Check sheet for the modelled part. Datum: model origin and axes. Units: mm. A direction names the side the tool comes from. Round coordinates to 2 decimals unless told otherwise and drop trailing zeros. Order: outer loops, then holes, each group sorted by start corner. A loop starts at its lowest first (then second) coordinate and runs counter-clockwise, first axis right, second up.
```python
from build123d import *

# Parameters (mm, degrees)
SKETCH_2_W           = 60
SKETCH_2_H           = 60
EXTRUDE_1_DEPTH      = 3
SKETCH_6_R           = 1.5
CUT_EXTRUDE_2_DEPTH  = 3
EXTRUDE_START        = -30
EXTRUDE_2_DEPTH      = 30
EXTRUDE_START_2      = 30
EXTRUDE_3_DEPTH      = 30
CUT_EXTRUDE_START    = 13
SKETCH_9_W           = 10
SKETCH_9_H           = 10
CUT_EXTRUDE_3_DEPTH  = 10
CUT_EXTRUDE_START_2  = -15
SKETCH_10_W          = 5
SKETCH_10_H          = 5
CUT_EXTRUDE_4_DEPTH  = 5
CUT_EXTRUDE_START_3  = 10
SKETCH_11_W          = 5
SKETCH_11_H          = 5
CUT_EXTRUDE_5_DEPTH  = 5
EXTRUDE_5_DEPTH      = 1.6
EXTRUDE_START_3      = -1.6
SKETCH_17_W          = 28
SKETCH_17_H          = 8
SKETCH_17_W_2        = 8
SKETCH_17_H_2        = 28
EXTRUDE_6_DEPTH      = 2
SKETCH_21_R          = 12.5
EXTRUDE_8_DEPTH      = 4
CUT_EXTRUDE_START_4  = -4
SKETCH_22_R          = 1.5
CUT_EXTRUDE_6_DEPTH  = 4
EXTRUDE_START_4      = -4
SKETCH_23_R          = 1.5
EXTRUDE_9_DEPTH      = 4
EXTRUDE_START_5      = -3.6
SKETCH_24_W          = 8
SKETCH_24_H          = 28
SKETCH_24_W_2        = 28
SKETCH_24_H_2        = 8
EXTRUDE_10_DEPTH     = 0.4
EXTRUDE_START_6      = 3
SKETCH_25_W          = 10
SKETCH_25_H          = 3
SKETCH_25_W_2        = 3
SKETCH_25_H_2        = 10
EXTRUDE_11_DEPTH     = 10
SKETCH_26_W          = 55
SKETCH_26_H          = 5
SKETCH_26_W_2        = 5
SKETCH_26_H_2        = 55
EXTRUDE_12_DEPTH     = 10
CUT_EXTRUDE_START_5  = -30
CUT_EXTRUDE_7_DEPTH  = 5
CUT_EXTRUDE_START_6  = 25
CUT_EXTRUDE_8_DEPTH  = 5
CUT_EXTRUDE_START_7  = 3
SKETCH_31_R          = 1
CUT_EXTRUDE_10_DEPTH = 3
CUT_EXTRUDE_11_DEPTH = 4
CUT_EXTRUDE_12_DEPTH = 13
SKETCH_34_W          = 20
SKETCH_34_H          = 20
CUT_EXTRUDE_14_DEPTH = 3
SKETCH_35_W          = 20
SKETCH_35_H          = 10
EXTRUDE_14_DEPTH     = 5
SKETCH_36_W          = 20
SKETCH_36_H          = 10
EXTRUDE_15_DEPTH     = 5
EXTRUDE_16_DEPTH     = 5
EXTRUDE_18_DEPTH     = 5
EXTRUDE_19_DEPTH     = 4
CUT_EXTRUDE_START_8  = -22
CUT_EXTRUDE_15_DEPTH = 44
CUT_EXTRUDE_16_DEPTH = 44
FILLET_1_R           = 5
FILLET_2_R           = 3


# Some blends are built 0.0001 mm under size
with BuildPart() as part:
    # 草图2 → 凸台-拉伸1 (new body)
    with BuildSketch(Plane(origin=(0, 0, 0), x_dir=(1, 0, 0), z_dir=(0, 1, 0))):
        Rectangle(SKETCH_2_W, SKETCH_2_H)
    extrude(amount=EXTRUDE_1_DEPTH)

    # 草图6 → 切除-拉伸2 (cut)
    with BuildSketch(Plane(origin=(0, 0, 0), x_dir=(1, 0, 0), z_dir=(0, 1, 0))):
        with Locations(Location((0, -7, 0), (0, 0, 270))):
            Circle(SKETCH_6_R)
        with Locations(Location((7, 0, 0), (0, 0, 270))):
            Circle(SKETCH_6_R)
        with Locations(Location((0, 7, 0), (0, 0, 270))):
            Circle(SKETCH_6_R)
        with Locations(Location((-7, 0, 0), (0, 0, 270))):
            Circle(SKETCH_6_R)
    extrude(amount=CUT_EXTRUDE_2_DEPTH, mode=Mode.SUBTRACT)

    # 草图7 → 凸台-拉伸2 (add)
    with BuildSketch(Plane.XY.offset(EXTRUDE_START)):
        Polygon((-15, 3), (-15, 8), (-20, 8), (-20, 13), (-10, 13), (-10, 3), align=None)
        Polygon((10, 3), (15, 3), (15, 8), (20, 8), (20, 13), (10, 13), align=None)
    extrude(amount=EXTRUDE_2_DEPTH)

    # 草图8 → 凸台-拉伸3 (add)
    with BuildSketch(Plane(origin=(0, 0, 0), x_dir=(0, 0, -1), z_dir=(1, 0, 0)).offset(EXTRUDE_START_2)):
        Polygon((-15, 3), (-15, 8), (-20, 8), (-20, 13), (-10, 13), (-10, 3), align=None)
        Polygon((10, 3), (15, 3), (15, 8), (20, 8), (20, 13), (10, 13), align=None)
    extrude(amount=-EXTRUDE_3_DEPTH)

    # 草图9 → 切除-拉伸3 (cut)
    with BuildSketch(Plane(origin=(0, 0, 0), x_dir=(1, 0, 0), z_dir=(0, 1, 0)).offset(CUT_EXTRUDE_START)):
        with Locations((25, 15)):
            Rectangle(SKETCH_9_W, SKETCH_9_H)
        with Locations((15, 25)):
            Rectangle(SKETCH_9_W, SKETCH_9_H)
    extrude(amount=-CUT_EXTRUDE_3_DEPTH, mode=Mode.SUBTRACT)

    # 草图10 → 切除-拉伸4 (cut)
    with BuildSketch(Plane.XY.offset(CUT_EXTRUDE_START_2)):
        with Locations((17.5, 5.5)):
            Rectangle(SKETCH_10_W, SKETCH_10_H)
    extrude(amount=CUT_EXTRUDE_4_DEPTH, mode=Mode.SUBTRACT)

    # 草图11 → 切除-拉伸5 (cut)
    with BuildSketch(Plane(origin=(0, 0, 0), x_dir=(0, 0, -1), z_dir=(1, 0, 0)).offset(CUT_EXTRUDE_START_3)):
        with Locations((17.5, 5.5)):
            Rectangle(SKETCH_11_W, SKETCH_11_H)
    extrude(amount=CUT_EXTRUDE_5_DEPTH, mode=Mode.SUBTRACT)

    # 草图16 → 凸台-拉伸5 (add)
    with BuildSketch(Plane(origin=(0, 0, 0), x_dir=(1, 0, 0), z_dir=(0, 1, 0))):
        Polygon((-10, -25), (15, -25), (15, -30), (18, -30), (18, -22), (-10, -22), align=None)
        Polygon((-22, 18), (-22, -10), (-25, -10), (-25, 15), (-30, 15), (-30, 18), align=None)
    extrude(amount=-EXTRUDE_5_DEPTH)

    # 草图17 → 凸台-拉伸6 (add)
    with BuildSketch(Plane(origin=(0, 0, 0), x_dir=(1, 0, 0), z_dir=(0, 1, 0)).offset(EXTRUDE_START_3)):
        with Locations((4, -26)):
            Rectangle(SKETCH_17_W, SKETCH_17_H)
        with Locations((-26, 4)):
            Rectangle(SKETCH_17_W_2, SKETCH_17_H_2)
    extrude(amount=-EXTRUDE_6_DEPTH)

    # 草图21 → 凸台-拉伸8 (add)
    with BuildSketch(Plane(origin=(0, 0, 0), x_dir=(1, 0, 0), z_dir=(0, 1, 0))):
        with Locations(Location((0, 0, 0), (0, 0, 270))):
            Circle(SKETCH_21_R)
    extrude(amount=-EXTRUDE_8_DEPTH)

    # 草图22 → 切除-拉伸6 (cut)
    with BuildSketch(Plane(origin=(0, 0, 0), x_dir=(1, 0, 0), z_dir=(0, 1, 0)).offset(CUT_EXTRUDE_START_4)):
        with Locations(Location((7, 0, 0), (0, 0, 270))):
            Circle(SKETCH_22_R)
        with Locations(Location((0, -7, 0), (0, 0, 270))):
            Circle(SKETCH_22_R)
        with Locations(Location((-7, 0, 0), (0, 0, 270))):
            Circle(SKETCH_22_R)
        with Locations(Location((0, 7, 0), (0, 0, 270))):
            Circle(SKETCH_22_R)
    extrude(amount=CUT_EXTRUDE_6_DEPTH, mode=Mode.SUBTRACT)

    # 草图23 → 凸台-拉伸9 (add)
    with BuildSketch(Plane(origin=(0, 0, 0), x_dir=(1, 0, 0), z_dir=(0, 1, 0)).offset(EXTRUDE_START_4)):
        Polygon((22, -18), (18, -22), (-10, -22), (-22, -10), (-22, 18), (-18, 22), (-18, 30), (18, 30), (18, 22), (22, 18), (30, 18), (30, -18), align=None)
        with Locations(Location((0, 7, 0), (0, 0, 270))):
            Circle(SKETCH_23_R, mode=Mode.SUBTRACT)
        with Locations(Location((7, 0, 0), (0, 0, 270))):
            Circle(SKETCH_23_R, mode=Mode.SUBTRACT)
        with Locations(Location((-7, 0, 0), (0, 0, 270))):
            Circle(SKETCH_23_R, mode=Mode.SUBTRACT)
        with Locations(Location((0, -7, 0), (0, 0, 270))):
            Circle(SKETCH_23_R, mode=Mode.SUBTRACT)
    extrude(amount=EXTRUDE_9_DEPTH)

    # 草图24 → 凸台-拉伸10 (add)
    with BuildSketch(Plane(origin=(0, 0, 0), x_dir=(1, 0, 0), z_dir=(0, 1, 0)).offset(EXTRUDE_START_5)):
        with Locations((-26, 4)):
            Rectangle(SKETCH_24_W, SKETCH_24_H)
        with Locations((4, -26)):
            Rectangle(SKETCH_24_W_2, SKETCH_24_H_2)
    extrude(amount=-EXTRUDE_10_DEPTH)

    # 草图25 → 凸台-拉伸11 (add)
    with BuildSketch(Plane(origin=(0, 0, 0), x_dir=(1, 0, 0), z_dir=(0, 1, 0)).offset(EXTRUDE_START_6)):
        with Locations((-15, -1.5)):
            Rectangle(SKETCH_25_W, SKETCH_25_H)
        with Locations((-1.5, -15)):
            Rectangle(SKETCH_25_W_2, SKETCH_25_H_2)
    extrude(amount=EXTRUDE_11_DEPTH)

    # 草图26 → 凸台-拉伸12 (add)
    with BuildSketch(Plane(origin=(0, 0, 0), x_dir=(1, 0, 0), z_dir=(0, 1, 0)).offset(EXTRUDE_START_6)):
        with Locations((2.5, -27.5)):
            Rectangle(SKETCH_26_W, SKETCH_26_H)
        with Locations((-27.5, 2.5)):
            Rectangle(SKETCH_26_W_2, SKETCH_26_H_2)
        with Locations((-27.5, -27.5)):
            Rectangle(SKETCH_26_W_2, SKETCH_26_H)
    extrude(amount=EXTRUDE_12_DEPTH)

    # 草图27 → 切除-拉伸7 (cut)
    with BuildSketch(Plane(origin=(0, 0, 0), x_dir=(0, 0, -1), z_dir=(1, 0, 0)).offset(CUT_EXTRUDE_START_5)):
        with BuildLine():
            Line((22.5, 6), (-22.5, 6))
            ThreePointArc((-22.5, 6), (-24.5, 8), (-22.5, 10))
            Line((-22.5, 10), (22.5, 10))
            ThreePointArc((22.5, 10), (24.5, 8), (22.5, 6))
        make_face()
    extrude(amount=CUT_EXTRUDE_7_DEPTH, mode=Mode.SUBTRACT)

    # 草图28 → 切除-拉伸8 (cut)
    with BuildSketch(Plane.XY.offset(CUT_EXTRUDE_START_6)):
        with BuildLine():
            Line((-22.5, 10), (22.5, 10))
            ThreePointArc((22.5, 10), (24.5, 8), (22.5, 6))
            Line((22.5, 6), (-22.5, 6))
            ThreePointArc((-22.5, 6), (-24.5, 8), (-22.5, 10))
        make_face()
    extrude(amount=CUT_EXTRUDE_8_DEPTH, mode=Mode.SUBTRACT)

    # 草图31 → 切除-拉伸10 (cut)
    with BuildSketch(Plane(origin=(0, 0, 0), x_dir=(1, 0, 0), z_dir=(0, 1, 0)).offset(CUT_EXTRUDE_START_7)):
        with Locations(Location((-20, -20, 0), (0, 0, 270))):
            Circle(SKETCH_31_R)
    extrude(amount=-CUT_EXTRUDE_10_DEPTH, mode=Mode.SUBTRACT)

    # 草图32 → 切除-拉伸11 (cut)
    with BuildSketch(Plane(origin=(0, 0, 0), x_dir=(1, 0, 0), z_dir=(0, 1, 0))):
        Polygon((30, 30), (30, 25), (25, 30), align=None)
    extrude(amount=CUT_EXTRUDE_11_DEPTH, mode=Mode.SUBTRACT)

    # 草图33 → 切除-拉伸12 (cut)
    with BuildSketch(Plane(origin=(0, 0, 0), x_dir=(1, 0, 0), z_dir=(0, 1, 0))):
        Polygon((-30, -30), (-27, -30), (-30, -27), align=None)
    extrude(amount=CUT_EXTRUDE_12_DEPTH, mode=Mode.SUBTRACT)

    # 草图34 → 切除-拉伸14 (cut)
    with BuildSketch(Plane(origin=(0, 0, 0), x_dir=(1, 0, 0), z_dir=(0, 1, 0)).offset(CUT_EXTRUDE_START_7)):
        Rectangle(SKETCH_34_W, SKETCH_34_H)
    extrude(amount=-CUT_EXTRUDE_14_DEPTH, mode=Mode.SUBTRACT)

    # 草图35 → 凸台-拉伸14 (add)
    with BuildSketch(Plane(origin=(0, 0, 0), x_dir=(0, 0, -1), z_dir=(1, 0, 0)).offset(EXTRUDE_START_2)):
        with Locations((0, 8)):
            Rectangle(SKETCH_35_W, SKETCH_35_H)
    extrude(amount=-EXTRUDE_14_DEPTH)

    # 草图36 → 凸台-拉伸15 (add)
    with BuildSketch(Plane.XY.offset(EXTRUDE_START)):
        with Locations((0, 8)):
            Rectangle(SKETCH_36_W, SKETCH_36_H)
    extrude(amount=EXTRUDE_15_DEPTH)

    # 草图37 → 凸台-拉伸16 (add)
    with BuildSketch(Plane.XY.offset(EXTRUDE_START)):
        Polygon((10, 3), (10, 13), (20, 13), (20, 8), (15, 8), (15, 3), align=None)
    extrude(amount=EXTRUDE_16_DEPTH)

    # 草图38 → 凸台-拉伸18 (add)
    with BuildSketch(Plane(origin=(0, 0, 0), x_dir=(0, 0, -1), z_dir=(1, 0, 0)).offset(EXTRUDE_START_2)):
        Polygon((10, 13), (20, 13), (20, 8), (15, 8), (15, 3), (10, 3), align=None)
    extrude(amount=-EXTRUDE_18_DEPTH)

    # 草图40 → 凸台-拉伸19 (add)
    with BuildSketch(Plane(origin=(0, 0, 0), x_dir=(1, 0, 0), z_dir=(0, 1, 0))):
        Polygon((-30, 18), (-18, 30), (-18, 22), (-22, 18), align=None)
        Polygon((18, 30), (30, 18), (22, 18), (18, 22), align=None)
        Polygon((30, -18), (18, -30), (18, -22), (22, -18), align=None)
    extrude(amount=-EXTRUDE_19_DEPTH)

    # 草图41 → 切除-拉伸15 (cut)
    with BuildSketch(Plane.XY.offset(CUT_EXTRUDE_START_8)):
        Polygon((30, 0), (26, -4), (30, -4), align=None)
    extrude(amount=CUT_EXTRUDE_15_DEPTH, mode=Mode.SUBTRACT)

    # 草图42 → 切除-拉伸16 (cut)
    with BuildSketch(Plane(origin=(0, 0, 0), x_dir=(0, 0, -1), z_dir=(1, 0, 0)).offset(CUT_EXTRUDE_START_8)):
        Polygon((30, -4), (30, 0), (26, -4), align=None)
    extrude(amount=CUT_EXTRUDE_16_DEPTH, mode=Mode.SUBTRACT)

    # 圆角1
    # the kernel refuses this fillet: 5 mm, written as the material it adds along each edge
    with BuildSketch(Plane(origin=(9.339745962, 0, -38.660254038), x_dir=(1.104671909501692e-12, -1.0, -1.104671909501665e-12), z_dir=(0.7071067811865389, 0, 0.7071067811865562))) as fillet_1_piece_1_section:
        with BuildLine():
            CenterArc((5, 4.898979486), FILLET_1_R, 180, 78.463040967)
            Line((0, 4.898979486), (-0.1, 4.898979486))
            Line((-0.1, 4.898979486), (-0.1, 0))
            Line((-0.1, 0), (0, -0.1))
            ThreePointArc((0, -0.1), (2, -0.1), (3.98, -0.09797959))
            Line((3.98, -0.09797959), (4, 0))
        make_face()
    fillet_1_piece_1 = extrude(amount=41.465460176, mode=Mode.PRIVATE)
    fillet_1_piece_1 = split(fillet_1_piece_1, bisect_by=Plane(origin=(24.77055683, -0.893670134, -30), z_dir=(0, 0, 1)), keep=Keep.TOP, mode=Mode.PRIVATE)
    fillet_1_piece_1 = split(fillet_1_piece_1, bisect_by=Plane(origin=(24.77055683, -3.061556652, -26.938443348), z_dir=(0, 0.7071067811865475, 0.7071067811865477)), keep=Keep.TOP, mode=Mode.PRIVATE)
    fillet_1_piece_1 = split(fillet_1_piece_1, bisect_by=Plane(origin=(26.938443348, -3.061556652, -24.77055683), z_dir=(-0.7071067811865591, 0.7071067811865359, 0)), keep=Keep.TOP, mode=Mode.PRIVATE)
    fillet_1_piece_1 = split(fillet_1_piece_1, bisect_by=Plane(origin=(30, -0.893670134, -24.77055683), z_dir=(-1, 0, 0)), keep=Keep.TOP, mode=Mode.PRIVATE)
    add(fillet_1_piece_1)

    # 圆角2
    fillet_2_edges = [part.edges().sort_by_distance(p)[0] for p in [
        (-6.5, 3, 10),
        (-10, 3, 6.5),
        (-5, 3, -10),
        (10, 3, 5),
    ]]
    fillet(fillet_2_edges, radius=FILLET_2_R - 0.0001)  # a hair under: the kernel refuses the full size


solid = part.part
```
Item 1: Release check for a two-part mould opening along Z. For faces 6 (the flat face through (-28, 6, 29)), 7 (the flat face through (12, 8, 10)), 8 (the flat face through (10, 7, -7)), 9 (the flat face through (0, 6, 27)) record: released by +Z, released by -Z, zero draft, split by the parting line, or undercut.
Answer:
face 6: released by +Z
face 7: undercut
face 8: undercut
face 9: zero draft
Item 2: Access from +Z, -Z, +X, -X, +Y, -Y to the whole of each face (thin tool, end or side, straight path). Record for faces 1 (the flat face through (-16, -2, 16)), 2 (the flat face through (20, 10, -10)), 3 (the flat face through (20, 11, -28)), 4 (the flat face through (-15, 8, 3)), 5 (the flat face through (10, 11, -20)).
Answer:
face 1: +Z, -X, -Y
face 2: -Z, +Y
face 3: -Z, +X, +Y
face 4: +Y
face 5: +X, +Y
Item 3: Scan lines: line 1 along X through (y, z) = (3.25, -3.5); line 2 along X through (y, z) = (-1.15, 0); line 3 along X through (y, z) = (-2.95, 0). Record each from-to range of solid material in increasing order.
Answer:
line 1: x = -30 to -25, -15 to -10, 10 to 15, 25 to 30
line 2: x = -25 to -8.5, -5.5 to 5.5, 8.5 to 28.85
line 3: x = -30 to -8.5, -5.5 to 5.5, 8.5 to 27.05
Item 4: Sectioned sample at D-D (x = -11.5). Record the cut outline in (y, z), and give its area (3 significant figures).
Answer:
outline: (-4, -26) - (0, -30) - (13, -30) - (13, 3) - (2.6, 3) - (2.6, 11.5) arc R3 ccw to (3, 13) - (3, 25) - (6, 25) - (6, 30) - (0, 30) - (0, 20.5) - (-4, 20.5) - close; (10, 25) - (13, 25) - (13, 30) - (10, 30) - close
area: 730 mm2
Item 5: Sectioned sample at A-A (x = 7). State how many separate pieces and enclosed holes the cut face has, and give its area (3 significant figures).
Answer:
separate pieces: 3
enclosed holes: 0
area: 562 mm2
Item 6: Go/stop test with flat-tipped pins: P1, Ø2.5, axis at y = 10.5, z = -28, coming from the +X side; P2, Ø2.5, axis at y = 4.5, z = 18, coming from the +X side; P3, Ø0.8, axis at x = -28.5, y = -0.5, coming from the +Z side. Record where each tip stops, or that it passes through.
Answer:
P1: stops at x = 20
P2: stops at x = 0
P3: stops at z = -15
Item 7: Sectioned sample at C-C (z = -16.5). Record the cut outline in (x, y).
Answer:
outline: (-30, -4) - (26, -4) - (30, 0) - (30, 3) - (-10, 3) - (-10, 13) - (-20, 13) - (-20, 8) - (-15, 8) - (-15, 3) - (-25, 3) - (-25, 6) - (-30, 6) - close; (-30, 10) - (-25, 10) - (-25, 13) - (-30, 13) - close; (0, 8) - (20, 8) - (20, 13) - (0, 13) - close; (25, 8) - (30, 8) - (30, 13) - (25, 13) - close
